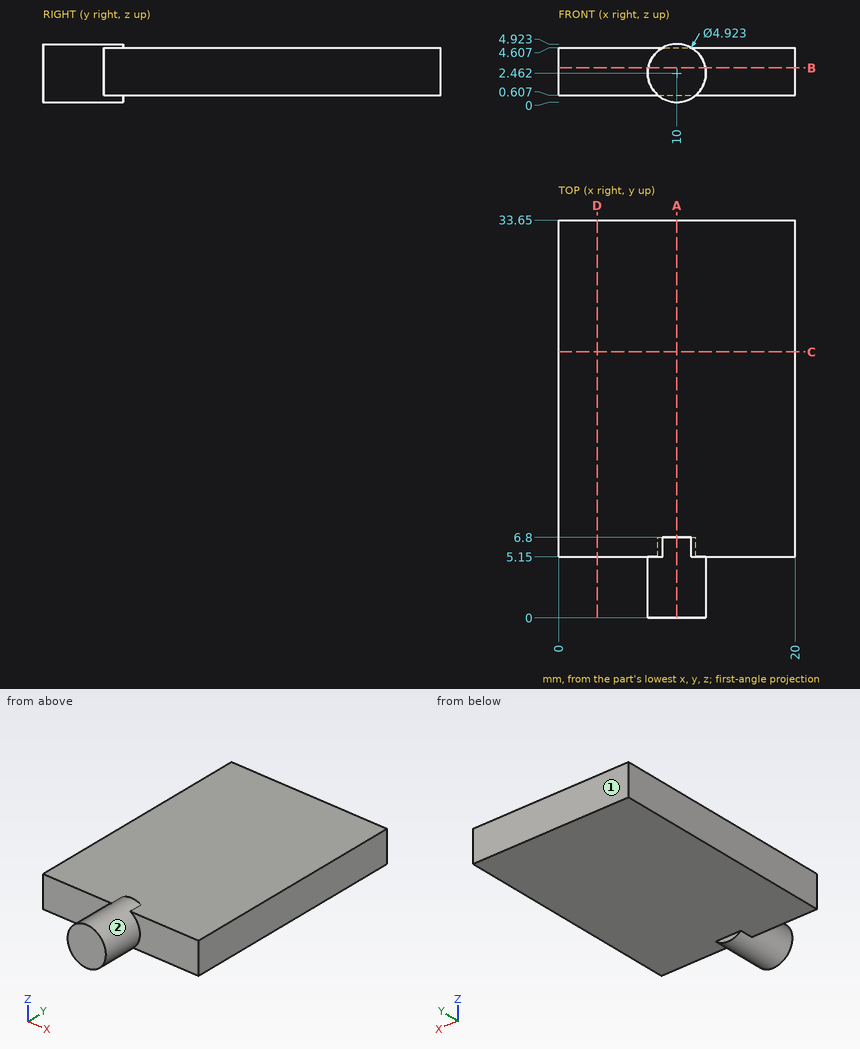
For this review, use the dimensioned drawing (mm, ordinates from the lowest corner) and the shaded views. A direction names the side the tool comes from. Round coordinates to 2 decimals unless told otherwise and drop trailing zeros. Order: outer loops, then holes, each group sorted by start corner. A loop starts at its lowest first (then second) coordinate and runs counter-clockwise, first axis right, second up.
1) For L1, parallel to Y at x = 1.75, z = 3; L2, parallel to Z at x = 2.25, y = 24; L3, parallel to Y at x = 10, z = 0.45, list the stretches that pass through material, from the lowest coordinate up.
The answers:
L1: y = 5.15 to 33.65
L2: z = 0.61 to 4.61
L3: y = 0 to 6.8
2) Machinability: for the marked faces 1 and 2, which of the approach directions +Z, -Z, +X, -X, +Y, -Y give a long, thin tool a straight path to every point of the face, cutting with its end or side? Answer none if there is none.
The answers:
face 1: +Z, -Z, +X, -X, +Y
face 2: -Y
3) Consider section A-A (x = 10). State the section outline as (y, z) points.
The answers:
outline: (0, 0) - (6.8, 0) - (6.8, 0.61) - (33.65, 0.61) - (33.65, 4.61) - (6.8, 4.61) - (6.8, 4.92) - (0, 4.92) - close
4) Consider section B-B (z = 2.9). State the section outline as (x, y) points, plus the area to 3 significant figures.
The answers:
outline: (0, 5.15) - (7.58, 5.15) - (7.58, 0) - (12.42, 0) - (12.42, 5.15) - (20, 5.15) - (20, 33.65) - (0, 33.65) - close
area: 595 mm2
5) Consider section C-C (y = 22.5). State the section outline as (x, z) points, plus the area to 3 significant figures.
The answers:
outline: (0, 0.61) - (20, 0.61) - (20, 4.61) - (0, 4.61) - close
area: 80.0 mm2
6) Clearance check with flat-ended pins moving along their axes: pin 1 Ø1 at (y, z) = (24.5, 4.5) entering from -X; pin 2 Ø6 at (x, y) = (12, 24) entering from +Z; pin 3 Ø2 at (x, z) = (3, 2.5) entering from -Y. State where each tip first meets the part, or that it passes through.
The answers:
pin 1: stops at x = 0
pin 2: stops at z = 4.61
pin 3: stops at y = 5.15
7) Consider section D-D (x = 3.25). State the section outline as (y, z) points.
The answers:
outline: (5.15, 0.61) - (33.65, 0.61) - (33.65, 4.61) - (5.15, 4.61) - close
